```python
from build123d import *

# Parameters (mm, degrees)
ESBO_O1_R                 = 8
ESBO_O1_R_2               = 4
RESSALTO_EXTRUS_O1_DEPTH  = 3
FURO_COM_FOLGA_DE_M1_61_D = 1.8
PADR_OCIRCULAR1_COUNT     = 6


with BuildPart() as part:
    # Esboço1 → Ressalto-extrusão1 (new body)
    with BuildSketch(Plane.XY):
        Circle(ESBO_O1_R)
        Circle(ESBO_O1_R_2, mode=Mode.SUBTRACT)
    extrude(amount=RESSALTO_EXTRUS_O1_DEPTH)

    # Furo com folga de M1.61 (through all)
    with Locations(Plane(origin=(0, 6, 3), x_dir=(1, 0, 0), z_dir=(0, 0, 1))):
        with Locations((0, 0)):
            furo_com_folga_de_m1_61 = Hole(FURO_COM_FOLGA_DE_M1_61_D / 2)

    # PadrãoCircular1: Furo com folga de M1.61 ×6 about axis
    padr_ocircular1_axis = Axis((0, 0, 0), (0, 0, 1))
    for i in range(1, PADR_OCIRCULAR1_COUNT):
        add(furo_com_folga_de_m1_61.rotate(padr_ocircular1_axis, i * 360 / PADR_OCIRCULAR1_COUNT), mode=Mode.SUBTRACT)


solid = part.part
```
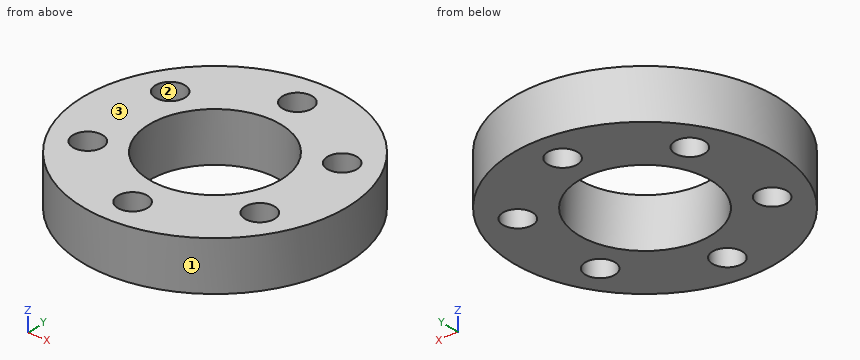
Work out the finished part from the listing and answer in its coordinate system (mm). Face numbers are marked on the shaded views. Round coordinates to 2 decimals unless told otherwise and drop trailing zeros. Loops run counter-clockwise (first coordinate to the right, second up) from the corner with the lowest first, then second, coordinate; pieces in that order, holes last.
(1) The part is cut by section A-A, the plane y = 0. Give the vertices of the cut face in (x, z), and give its area (3 significant figures).
Computed values:
outline: (-8, 0) - (-4, 0) - (-4, 3) - (-8, 3) - close; (4, 0) - (8, 0) - (8, 3) - (4, 3) - close
area: 24.0 mm2
(2) The part is cut by section D-D, the plane x = 4.5. Give the vertices of the cut face in (y, z), and give its area (3 significant figures).
Computed values:
outline: (-6.61, 0) - (-3.57, 0) - (-3.57, 3) - (-6.61, 3) - close; (-2.43, 0) - (2.43, 0) - (2.43, 3) - (-2.43, 3) - close; (3.57, 0) - (6.61, 0) - (6.61, 3) - (3.57, 3) - close
area: 32.8 mm2
(3) The mould has two halves that part along X. Classify the marked faces 1, 2 and 3: pulls with the +X half, pulls with the -X half, needs draft (parallel to the pull), parting line crosses it, or undercut.
Computed values:
face 1: parting line crosses it
face 2: undercut
face 3: needs draft
(4) The part is cut by section C-C, the plane z = 2.8. Give the vertices of the cut face in (x, y), and give its area (3 significant figures).
Computed values:
outline: circle Ø16 at (0, 0); hole circle Ø1.8 at (-5.2, -3); hole circle Ø1.8 at (-5.2, 3); hole circle Ø8 at (0, 0); hole circle Ø1.8 at (0, -6); hole circle Ø1.8 at (0, 6); hole circle Ø1.8 at (5.2, -3); hole circle Ø1.8 at (5.2, 3)
area: 136 mm2
(5) Find the intervals of material crossed by L1, parallel to Y at x = 0, z = 2.15; L2, parallel to X at y = 2.5, z = 2.55; L3, parallel to X at y = -3.5, z = 0.4, in increasing order.
Computed values:
L1: y = -8 to -6.9, -5.1 to -4, 4 to 5.1, 6.9 to 8
L2: x = -7.6 to -5.94, -4.45 to -3.12, 3.12 to 4.45, 5.94 to 7.6
L3: x = -7.19 to -5.94, -4.45 to -1.94, 1.94 to 4.45, 5.94 to 7.19
(6) The part is cut by section B-B, the plane x = 0. Give the vertices of the cut face in (y, z), and give its area (3 significant figures).
Computed values:
outline: (-8, 0) - (-6.9, 0) - (-6.9, 3) - (-8, 3) - close; (-5.1, 0) - (-4, 0) - (-4, 3) - (-5.1, 3) - close; (4, 0) - (5.1, 0) - (5.1, 3) - (4, 3) - close; (6.9, 0) - (8, 0) - (8, 3) - (6.9, 3) - close
area: 13.2 mm2
(7) This flat-tipped pin is pushed along its axis until it touches: P1, Ø1.5, axis at y = -1.5, z = 0.5, coming from the -X side. Where does it stop, or does it pass through?
Computed values:
P1: stops at x = -7.96
